Autodesk Inventor part; units mm, degrees
ref_plane "YZ Plane" through (0, 0, 0) normal (1, 0, 0) x (0, 1, 0)
ref_plane "XZ Plane" through (0, 0, 0) normal (0, 1, 0) x (-1, 0, 0)
ref_plane "XY Plane" through (0, 0, 0) normal (0, 0, 1) x (1, 0, 0)
sketch "Sketch1" plane through (0, 0, 0) normal (0, 1, 0) x (-1, 0, 0)
  line L0 (-22.5, 22.5) -> (22.5, 22.5)
  line L1 (22.5, 22.5) -> (22.5, -22.5)
  line L2 (22.5, -22.5) -> (-22.5, -22.5)
  line L3 (-22.5, -22.5) -> (-22.5, 22.5)
  line L4 (-22.5, 22.5) -> (22.5, -22.5) construction
  line L5 (22.5, 22.5) -> (-22.5, -22.5) construction
  circle A0 centre (0, 0) radius 20
  dimension "d0" = 40
  dimension "d1" = 45
  dimension "d2" = 45
extrude "Extrusion1" add sketch "Sketch1" along normal blind 8
sketch "Sketch2" plane through (22.5, 0, -22.5) normal (0, 0, -1) x (-1, 0, 0)
  line L0 (0, 0) -> (45, 0)
  line L1 (45, 0) -> (0, 0)
  line L2 (0, 0) -> (0, 30)
  line L3 (0, 30) -> (45, 30)
  line L4 (45, 30) -> (45, 0)
  line L5 (45, 0) -> (0, 0)
  line L6 (0, 0) -> (0, -45)
  line L7 (0, -45) -> (45, -45)
  line L8 (45, -45) -> (45, 0)
  point P0 (22.5, 0)
  dimension "d5" = 30
  dimension "d8" = 45
extrude "Extrusion2" add sketch "Sketch2" along normal blind 8
chamfer "Chamfer1" distance 2 angle 45 2 edges at (0, 8, -22.5) (0, 0, -22.5)
properties part number "Air Filter Bracket" material "Acetal Resin, White"
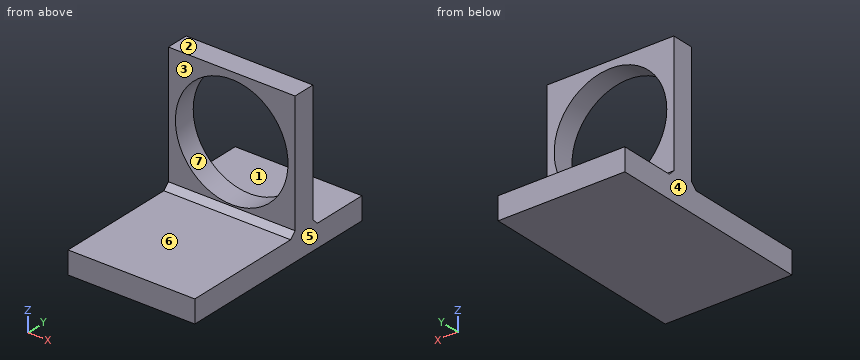
Verification items for the finished model (mm, model axes). Face numbers are marked on the shaded views. A direction names the side the tool comes from. Coordinates: 2 decimals unless noted, no trailing zeros. Loops run counter-clockwise (first coordinate to the right, second up) from the corner with the lowest first, then second, coordinate; pieces in that order, holes last. Notation, with made-up numbers: M 67,33 L 112,33 A20 ccw 112,56 Z; hole C 53,36 d8. An arc over 180 degrees is marked long. One line per item, written item: value.
1. Material ranges on line 1 along Z through (x, y) = (0, 5); line 2 along Z through (x, y) = (-8.5, 19); line 3 along Y through (x, z) = (-20, -20.5), recorded low to high. Write a range as from..to.
Answers follow:
line 1: -30.5..-20, 20..22.5
line 2: -30.5..-22.5
line 3: 0..8
2. Gauge pin test, flat ends, axial feed: P1, Ø16, axis at x = -6, y = 21, coming from the +Z side; P2, Ø21.5, axis at x = 2.5, z = 5.5, coming from the +Y side; P3, Ø6, axis at x = 17, z = -8, coming from the -Y side. Record the tip position at first contact, or that the pin passes through.
Answers follow:
P1: z = -22.5
P2: through
P3: y = 0
3. Section check C-C on z = 12. Record the cut outline in (x, y).
Answers follow:
outline: M -22.5,0 L -16,0 L -16,8 L -22.5,8 Z; M 16,0 L 22.5,0 L 22.5,8 L 16,8 Z
4. Mould release check, pull along X, two halves, no side actions. Record for the marked faces 4, 5, 6 and 7: pulls with the +X half, pulls with the -X half, needs draft (parallel to the pull), parting line crosses it, or undercut.
Answers follow:
face 4: pulls with the -X half
face 5: pulls with the +X half
face 6: needs draft
face 7: undercut
5. Set-up check for the marked faces 1, 2 and 3: record each of +Z, -Z, +X, -X, +Y, -Y from which the full face is reachable in a straight line by a thin tool's end or side.
Answers follow:
face 1: +Z, +X, -X, +Y
face 2: +Z, +X, -X, +Y, -Y
face 3: +Z, +X, -X, -Y
6. Section check D-D on x = 0. Record the cut outline in (y, z).
Answers follow:
outline: M -45,-30.5 L 30,-30.5 L 30,-22.5 L 10,-22.5 L 8,-20.5 L 8,-20 L 0,-20 L 0,-20.5 L -2,-22.5 L -45,-22.5 Z; M 0,20 L 8,20 L 8,22.5 L 0,22.5 Z
7. Section check A-A on z = 0. Record the cut outline in (x, y).
Answers follow:
outline: M -22.5,0 L -20,0 L -20,8 L -22.5,8 Z; M 20,0 L 22.5,0 L 22.5,8 L 20,8 Z
8. Section check B-B on x = -4.5. Record the cut outline in (y, z).
Answers follow:
outline: M -45,-30.5 L 30,-30.5 L 30,-22.5 L 10,-22.5 L 8,-20.5 L 8,-19.49 L 0,-19.49 L 0,-20.5 L -2,-22.5 L -45,-22.5 Z; M 0,19.49 L 8,19.49 L 8,22.5 L 0,22.5 Z
